```python
from build123d import *

# Parameters (mm, degrees)
SKETCH1_R           = 3.885
SKETCH1_R_2         = 1.59
BOSS_EXTRUDE1_DEPTH = 3.75
CHAMFER1_SIZE       = 0.6
CUT_EXTRUDE1_DEPTH  = 3.75


with BuildPart() as part:
    # Sketch1 → Boss-Extrude1 (new body)
    with BuildSketch(Plane.XY):
        Circle(SKETCH1_R)
        Circle(SKETCH1_R_2, mode=Mode.SUBTRACT)
    extrude(amount=BOSS_EXTRUDE1_DEPTH)

    # Chamfer1
    chamfer1_edges = [part.edges().sort_by_distance(p)[0] for p in [
        (-3.885, 0, 0),
        (-3.885, 0, 3.75),
    ]]
    chamfer(chamfer1_edges, length=CHAMFER1_SIZE)

    # Sketch2 → Cut-Extrude1 (cut)
    with BuildSketch(Plane(origin=(0, 0, 0), x_dir=(-1, 0, 0), z_dir=(0, 0, -1))):
        with BuildLine():
            Line((-3.883814063, -0.09598607), (-2.025033407, 3.315488607))
            ThreePointArc((-2.025033407, 3.315488607), (-3.411474677, 1.858780656), (-3.883814063, -0.09598607))
        make_face()
        with BuildLine():
            Line((-1.858780656, -3.411474677), (-3.883814063, -0.09598607))
            ThreePointArc((-3.883814063, -0.09598607), (-3.315488607, -2.025033407), (-1.858780656, -3.411474677))
        make_face()
        with BuildLine():
            ThreePointArc((-1.858780656, -3.411474677), (0.09598607, -3.883814063), (2.025033407, -3.315488607))
            Line((2.025033407, -3.315488607), (-1.858780656, -3.411474677))
        make_face()
        with BuildLine():
            ThreePointArc((3.885, 0), (3.884703504, 0.047996698), (3.883814063, 0.09598607))
            Line((3.883814063, 0.09598607), (2.025033407, -3.315488607))
            ThreePointArc((2.025033407, -3.315488607), (3.38825027, -1.900785392), (3.885, 0))
        make_face()
        with BuildLine():
            ThreePointArc((3.883814063, 0.09598607), (3.315488607, 2.025033407), (1.858780656, 3.411474677))
            Line((1.858780656, 3.411474677), (3.883814063, 0.09598607))
        make_face()
        with BuildLine():
            Line((-2.025033407, 3.315488607), (1.858780656, 3.411474677))
            ThreePointArc((1.858780656, 3.411474677), (-0.09598607, 3.883814063), (-2.025033407, 3.315488607))
        make_face()
    extrude(amount=-CUT_EXTRUDE1_DEPTH, mode=Mode.SUBTRACT)


solid = part.part
```
Verification items for the finished model (mm, model axes). Give positions to 0.01 mm unless a question says otherwise; leave off trailing zeros. Loops run counter-clockwise (first coordinate to the right, second up) from the corner with the lowest first, then second, coordinate; pieces in that order, holes last.
1. Section check A-A, the plane z = 2.2. Enter the section's corners in (x, y), then the cut area to 3 significant figures.
2. Go/stop test with a flat-tipped pin: pin 1 Ø1 at (x, z) = (-3, 0.5) entering from +Y. Record where the tip stops, or that it passes through.
3. Section check B-B, the plane y = 0. Enter the section's corners in (x, z) (3 decimals).
4. Thickness scan on line 1 (Y direction, x = -0.75, z = 0.2); line 2 (Y direction, x = 0.75, z = 1.05); line 3 (X direction, y = 1, z = 1.8). Record the ranges inside material, lowest first.
5. Mould release check, pull along X, two halves, no side actions. Record for faces 1 (the flat face through (-2.967, -1.586, 1.85)), 2 (the cylindrical face through (-0.345, -1.552, 1.849)), 3 (the flat face through (-2, -1, 0)): released by +X, released by -X, zero draft, split by the parting line, or undercut.
6. Section check C-C, the plane x = 0. Enter the section's corners in (y, z) (3 decimals).
Geometry says:
1. outline: (-3.88, 0.1) - (-2.03, -3.32) - (1.86, -3.41) - (3.88, -0.1) - (2.03, 3.32) - (-1.86, 3.41) - close; hole circle Ø3.18 at (0, 0)
1. area: 31.3 mm2
2. pin 1: stops at y = 2.36
3. outline: (-3.832, 0.547) - (-3.285, 0) - (-1.59, 0) - (-1.59, 3.75) - (-3.285, 3.75) - (-3.832, 3.203) - close; (1.59, 0) - (3.285, 0) - (3.832, 0.547) - (3.832, 3.203) - (3.285, 3.75) - (1.59, 3.75) - close
4. line 1: y = -3.35 to -1.4, 1.4 to 3.38
4. line 2: y = -3.38 to -1.4, 1.4 to 3.35
4. line 3: x = -3.33 to -1.24, 1.24 to 3.29
5. face 1: released by -X
5. face 2: undercut
5. face 3: zero draft
6. outline: (-3.366, 0.081) - (-3.285, 0) - (-1.59, 0) - (-1.59, 3.75) - (-3.285, 3.75) - (-3.366, 3.669) - close; (1.59, 0) - (3.285, 0) - (3.366, 0.081) - (3.366, 3.669) - (3.285, 3.75) - (1.59, 3.75) - close
